Input: part model. Units: mm. Frame: model coordinates. A direction names the side the tool comes from. Give positions to 0.01 mm unless a question says otherwise; leave off trailing zeros. Loops run counter-clockwise (first coordinate to the right, second up) from the corner with the lowest first, then second, coordinate; pieces in that order, holes last. Notation, with made-up numbers: (85.25, -22.75) -> (136.25, -22.75) arc R32 ccw to (136.25, 12.25) -> close; hole circle Ø9 at (65, 24). An arc over 180 degrees is marked (long way). Answer as a JSON object with one key per item and string values.
```python
from build123d import *

# Parameters (mm, degrees)
SKETCH_1_R      = 1.5
EXTRUDE_1_DEPTH = 15
FILLET_1_R      = 5
FILLET_2_R      = 3


with BuildPart() as part:
    # 草图1 → 凸台-拉伸1 (new body)
    with BuildSketch(Plane.XY):
        Polygon((19.5, 9.5), (-19.5, 9.5), (-15, -11.5), (15, -11.5), align=None)
        with Locations((14, -5.5)):
            Circle(SKETCH_1_R, mode=Mode.SUBTRACT)
        with Locations((-14, -5.5)):
            Circle(SKETCH_1_R, mode=Mode.SUBTRACT)
        with Locations((-14, 5.5)):
            Circle(SKETCH_1_R, mode=Mode.SUBTRACT)
        with Locations((14, 5.5)):
            Circle(SKETCH_1_R, mode=Mode.SUBTRACT)
        Polygon((-12.078076687, 3.5), (-10.149505259, -5.5), (10.149505259, -5.5), (12.078076687, 3.5), align=None, mode=Mode.SUBTRACT)
    extrude(amount=EXTRUDE_1_DEPTH)

    # 圆角1
    fillet_1_edges = [part.edges().sort_by_distance(p)[0] for p in [
        (15, -11.5, 7.5),
        (-15, -11.5, 7.5),
        (-19.5, 9.5, 7.5),
        (19.5, 9.5, 7.5),
    ]]
    fillet(fillet_1_edges, radius=FILLET_1_R)

    # 圆角2
    fillet_2_edges = [part.edges().sort_by_distance(p)[0] for p in [
        (12.078076687, 3.5, 7.5),
        (-12.078076687, 3.5, 7.5),
        (-10.149505259, -5.5, 7.5),
        (10.149505259, -5.5, 7.5),
    ]]
    fillet(fillet_2_edges, radius=FILLET_2_R)


solid = part.part
```
Q1. Access query for faces 1 (the cylindrical face through (14.138, -10.358, 7.605)), 2 (the flat face through (-10.984, -1.608, 7.395)). Directions: +Z, -Z, +X, -X, +Y, -Y. A direction counts if a zero-diameter tool reaches every point of the face in a straight line with its end or side. Return the directions, or none.
Evaluation:
{"face 1": "+Z, -Z, +X, -Y", "face 2": "+Z, -Z"}
Q2. Draft query along Y for faces 3 (the flat face through (0, 4, 15)), 4 (the flat face through (-17.042, -1.971, 7.395)), 5 (the cylindrical face through (9.59, -4.85, 7.6)), 6 (the flat face through (0, 9.5, 7)). Return one class per face: +Y half, -Y half, draft (parallel to the pull), parting line (faces both ways), or undercut.
Evaluation:
{"face 3": "draft", "face 4": "-Y half", "face 5": "undercut", "face 6": "+Y half"}
Q3. Ray query, line 1 along Y through (x, z) = (-14, 11.5); line 2 along Y through (x, z) = (3, 9.25); line 3 along X through (y, z) = (-5.75, 10.25). Return the intervals inside material, ascending.
Evaluation:
{"line 1": "y = -10.47 to -7, -4 to 4, 7 to 9.45", "line 2": "y = -11.5 to -5.5, 3.5 to 9.5", "line 3": "x = -16.23 to -15.48, -12.52 to 12.52, 15.48 to 16.23"}
Q4. Section C-C, the plane y = 3. Return the cut outline in (x, z), then the cut area to 3 significant figures.
Evaluation:
{"outline": "(-18.11, 0) -> (-10.03, 0) -> (-10.03, 15) -> (-18.11, 15) -> close; (10.03, 0) -> (18.11, 0) -> (18.11, 15) -> (10.03, 15) -> close", "area": "242 mm2"}
Q5. Section B-B, the plane z = 10.25. Return the cut outline in (x, y).
Evaluation:
{"outline": "(-18.2, 3.45) -> (-15.85, -7.55) arc R5 ccw to (-10.96, -11.5) -> (10.96, -11.5) arc R5 ccw to (15.85, -7.55) -> (18.2, 3.45) arc R5 ccw to (13.32, 9.5) -> (-13.32, 9.5) arc R5 ccw to start; hole circle Ø3 at (-14, -5.5); hole circle Ø3 at (-14, 5.5); hole (-11.3, -0.13) -> (-10.66, -3.13) arc R3 ccw to (-7.72, -5.5) -> (7.72, -5.5) arc R3 ccw to (10.66, -3.13) -> (11.3, -0.13) arc R3 ccw to (8.37, 3.5) -> (-8.37, 3.5) arc R3 ccw to start; hole circle Ø3 at (14, -5.5); hole circle Ø3 at (14, 5.5)"}
Q6. Section A-A, the plane x = -6. Return the cut outline in (y, z).
Evaluation:
{"outline": "(-11.5, 0) -> (-5.5, 0) -> (-5.5, 15) -> (-11.5, 15) -> close; (3.5, 0) -> (9.5, 0) -> (9.5, 15) -> (3.5, 15) -> close"}
Q7. Pin query (flat end, axial travel): pin 1 (2 mm diameter, centred on y = 1.5, z = 9.5, fed in from +X); pin 2 (1.5 mm diameter, centred on x = -5.5, y = 5.5, fed in from -Z); pin 3 (4 mm diameter, centred on y = -0.5, z = 3.5, fed in from -X). Return the tip coordinate at first contact, or that it passes through.
Evaluation:
{"pin 1": "stops at x = 18", "pin 2": "stops at z = 0", "pin 3": "stops at x = -17.79"}
Q8. Section D-D, the plane x = 14. Return the cut outline in (y, z).
Evaluation:
{"outline": "(-10.47, 0) -> (-7, 0) -> (-7, 15) -> (-10.47, 15) -> close; (-4, 0) -> (4, 0) -> (4, 15) -> (-4, 15) -> close; (7, 0) -> (9.45, 0) -> (9.45, 15) -> (7, 15) -> close"}
